For this review, take the finished solid that the model builds, in its own axes (mm). Give positions to 0.01 mm unless a question says otherwise; leave off trailing zeros. Loops run counter-clockwise (first coordinate to the right, second up) from the corner with the lowest first, then second, coordinate; pieces in that order, holes last.
```python
from build123d import *

# Parameters (mm, degrees)
F0_W          = 105.8753505349
F0_H          = 70.4643428326
F1_DEPTH      = 25.4
F2_R          = 20.5218866045
F3_DEPTH      = 25.4
F5_DEPTH      = 35.2331714163
F5_DEPTH_BACK = 35.2331714163


with BuildPart() as f1:
    # F0 (on Top) → F1 (new body)
    with BuildSketch(Plane.XY):
        Rectangle(F0_W, F0_H)
    extrude(amount=F1_DEPTH)

    # F2 (on face) → F3 (join)
    with BuildSketch(Plane.XY.offset(25.4)):
        Circle(F2_R)
    extrude(amount=F3_DEPTH)

    # F4 (on Front) → F5 (cut, two sides)
    with BuildSketch(Plane.XZ) as f5_sk:
        Polygon((20.5218866045, 50.8), (-20.5218866045, 50.8), (20.5218866045, 25.4), align=None)
    extrude(amount=-F5_DEPTH, mode=Mode.SUBTRACT)
    extrude(f5_sk.sketch, amount=F5_DEPTH_BACK, mode=Mode.SUBTRACT)


solid = f1.part
```
Item 1: Take a section at A-A on x = 0. Give the boundary of the cut face in (y, z).
Answer:
outline: (-35.23, 0) - (35.23, 0) - (35.23, 25.4) - (20.52, 25.4) - (20.52, 38.1) - (-20.52, 38.1) - (-20.52, 25.4) - (-35.23, 25.4) - close
Item 2: Take a section at B-B on y = 17.5. Give the boundary of the cut face in (x, z), and give its area (3 significant figures).
Answer:
outline: (-52.94, 0) - (52.94, 0) - (52.94, 25.4) - (10.72, 25.4) - (10.72, 31.47) - (-10.72, 44.73) - (-10.72, 25.4) - (-52.94, 25.4) - close
area: 2,960 mm2
Item 3: Clearance check with flat-ended pins moving along their axes: pin 1 Ø12 at (x, y) = (21, 18.5) entering from +Z; pin 2 Ø1 at (y, z) = (7.5, 29.5) entering from +X; pin 3 Ø1 at (x, y) = (-11, 10) entering from +Z. State where each tip first meets the part, or that it passes through.
Answer:
pin 1: stops at z = 25.4
pin 2: stops at x = 14.7
pin 3: stops at z = 45.22
Item 4: For L1, parallel to Z at x = -35.5, y = -14.5; L2, parallel to X at y = -8.5, z = 45; L3, parallel to X at y = -5, z = 34.5, list the stretches that pass through material, from the lowest coordinate up.
Answer:
L1: z = 0 to 25.4
L2: x = -18.68 to -11.15
L3: x = -19.9 to 5.82
Item 5: Take a section at C-C on z = 39. Give the boundary of the cut face in (x, y), and give its area (3 significant figures).
Answer:
outline: (-1.45, -20.47) - (-1.45, 20.47) arc R20.52 ccw to start
area: 602 mm2
Item 6: Take a section at D-D on y = 27. Give the boundary of the cut face in (x, z), and give its area (3 significant figures).
Answer:
outline: (-52.94, 0) - (52.94, 0) - (52.94, 25.4) - (-52.94, 25.4) - close
area: 2,690 mm2
